Could you check a few things on this model? Use its own coordinates, in mm. A direction names the side the tool comes from. Give positions to 0.01 mm unless a question says otherwise; leave off trailing zeros. Loops run counter-clockwise (first coordinate to the right, second up) from the corner with the lowest first, then second, coordinate; pieces in that order, holes last. Notation, with made-up numbers: (27.25, 60.5) - (83.25, 60.5) arc R14 cw to (83.25, 75.5) - close; hole circle Ø7 at (89.25, 6.5). An arc over 180 degrees is marked (long way). Use CSV: the item, a comma, the result in double quotes.
from build123d import *

# Parameters (mm, degrees)
F2_R     = 4
F3_DEPTH = 25


with BuildPart() as f1:
    # F0 (on Front) → F1 (revolve)
    with BuildSketch(Plane.XZ):
        Polygon((0, 0), (0, 70), (-30, 70), (-13.895227, 47), (-13.895227, 38), (-29.551464, 9), (-41.551464, 9), (-41.551464, 18), (-51.551464, 18), (-45, 0), align=None)
    revolve(axis=Axis((0, 0, 35), (0, 0, 1)))

    # F2 (on face) → F3 (cut)
    with BuildSketch(Plane.XY.offset(9)):
        with Locations((-36, 0)):
            Circle(F2_R)
        with Locations((-18, -31.176915)):
            Circle(F2_R)
        with Locations((18, -31.176915)):
            Circle(F2_R)
        with Locations((36, 0)):
            Circle(F2_R)
        with Locations((18, 31.176915)):
            Circle(F2_R)
        with Locations((-18, 31.176915)):
            Circle(F2_R)
    extrude(amount=-F3_DEPTH, mode=Mode.SUBTRACT)


solid = f1.part
1) I'm going to push flat-ended pins straight in: P1, Ø4, axis at x = 31, y = 26.5, coming from the -Z side; P2, Ø5, axis at x = 26.5, z = 11.5, coming from the +Y side; P3, Ø7, axis at x = 18, y = -31.18, coming from the -Z side; P4, Ø1.5, axis at x = 38, y = 6.5, coming from the +Z side. Where does each tip first touch, or does it pass through?
Answer below:
P1,"stops at z = 0"
P2,"stops at y = 43.28"
P3,"passes through"
P4,"stops at z = 9"
2) Which directions (+Z, -Z, +X, -X, +Y, -Y) give clear straight access to the entire face, cutting with the end or side of a thin tool? Please do faces 4 (the cylindrical face through (3.012, 13.565, 42.437)), 5 (the cylindrical face through (32.974, 25.283, 13.563)), 6 (the flat face through (0, 0, 70)).
Answer below:
face 4,"none"
face 5,"+Z"
face 6,"+Z, +X, -X, +Y, -Y"
3) I need wall thicknesses on line 1 along Y through (x, z) = (7, 11.5) (3 decimals); line 2 along Y through (x, z) = (-18, 5); line 3 along X through (y, z) = (-33.5, 4.5). Which ranges of each line are inside material? Lowest first, please.
Answer below:
line 1,"y = -48.685 to -40.958, -27.319 to 27.319, 40.958 to 48.685"
line 2,"y = -43.22 to -35.18, -27.18 to 27.18, 35.18 to 43.22"
line 3,"x = -32.45 to -21.26, -14.74 to 14.74, 21.26 to 32.45"
4) Suppose I cut it at A-A (y = 0). Please give me the cut outline in (x, z).
Answer below:
outline,"(-51.55, 18) - (-45, 0) - (-40, 0) - (-40, 9) - (-41.55, 9) - (-41.55, 18) - close; (-32, 0) - (32, 0) - (32, 9) - (29.55, 9) - (13.9, 38) - (13.9, 47) - (30, 70) - (-30, 70) - (-13.9, 47) - (-13.9, 38) - (-29.55, 9) - (-32, 9) - close; (40, 0) - (45, 0) - (51.55, 18) - (41.55, 18) - (41.55, 9) - (40, 9) - close"
5) Suppose I cut it at B-B (x = 0). Please give me the cut outline in (y, z), plus the area to 3 significant figures.
Answer below:
outline,"(-51.55, 18) - (-45, 0) - (45, 0) - (51.55, 18) - (41.55, 18) - (41.55, 9) - (29.55, 9) - (13.9, 38) - (13.9, 47) - (30, 70) - (-30, 70) - (-13.9, 47) - (-13.9, 38) - (-29.55, 9) - (-41.55, 9) - (-41.55, 18) - close"
area,"3,510 mm2"
6) Suppose I cut it at C-C (x = 20). State how many separate pieces and enclosed holes the cut face has, plus the area to 3 significant figures.
Answer below:
separate pieces,"4"
enclosed holes,"0"
area,"1,700 mm2"
7) Suppose I cut it at D-D (z = 42). Please give me the cut outline in (x, y), plus the area to 3 significant figures.
Answer below:
outline,"circle Ø27.79 at (0, 0)"
area,"607 mm2"
8) We'd pull the mould along X, two halves only. Please class faces 1 (the cylindrical face through (-39.2, -2.4, 4.6)), 2 (the flat face through (-35, -23, 18)), 3 (the conical face through (3.18, 14.33, 48.12)): +X half, -X half, draft (parallel to the pull), parting line (faces both ways), or undercut.
Answer below:
face 1,"undercut"
face 2,"draft"
face 3,"parting line"
